from build123d import *

# Parameters (mm, degrees)
SKETCH1_R           = 60
SKETCH1_R_2         = 43.5
EXTRUSION1_DEPTH    = 60
EXTRUSION3_START    = -60
EXTRUSION3_DEPTH    = 60
BOSS_EXTRUDE1_START = -60
BOSS_EXTRUDE1_DEPTH = 60


with BuildPart() as part:
    # Sketch1 → Extrusion1 (new body)
    with BuildSketch(Plane.XY):
        Circle(SKETCH1_R)
        Circle(SKETCH1_R_2, mode=Mode.SUBTRACT)
    extrude(amount=EXTRUSION1_DEPTH)

    # Sketch3 → Extrusion3 (cut)
    with BuildSketch(Plane.XY.offset(60).offset(EXTRUSION3_START)):
        with BuildLine():
            Line((-0.5, 48.5), (-0.5, 43.497126342))
            ThreePointArc((-0.5, 43.497126342), (0, 43.5), (0.5, 43.497126342))
            Line((0.5, 43.497126342), (0.5, 48.5))
            Line((0.5, 48.5), (-0.5, 48.5))
        make_face()
    extrude(amount=EXTRUSION3_DEPTH, mode=Mode.SUBTRACT)

    # Sketch4 → Boss-Extrude1 (add)
    with BuildSketch(Plane.XY.offset(60).offset(BOSS_EXTRUDE1_START)):
        with BuildLine():
            Line((31.28966164, 51.195283713), (31.299038106, 51.211524227))
            Line((31.299038106, 51.211524227), (33.799038106, 55.541651246))
            Line((33.799038106, 55.541651246), (31.200961894, 57.041651246))
            Line((31.200961894, 57.041651246), (28.700961894, 52.711524227))
            Line((28.700961894, 52.711524227), (28.691585429, 52.695283713))
            ThreePointArc((28.691585429, 52.695283713), (30, 51.961524227), (31.28966164, 51.195283713))
        make_face()
        with BuildLine():
            Line((1.5, 59.981247069), (1.5, 60))
            Line((1.5, 60), (1.5, 65))
            Line((1.5, 65), (-1.5, 65))
            Line((-1.5, 65), (-1.5, 60))
            Line((-1.5, 60), (-1.5, 59.981247069))
            ThreePointArc((-1.5, 59.981247069), (0, 60), (1.5, 59.981247069))
        make_face()
        with BuildLine():
            Line((52.695283713, 28.691585429), (52.711524227, 28.700961894))
            Line((52.711524227, 28.700961894), (57.041651246, 31.200961894))
            Line((57.041651246, 31.200961894), (55.541651246, 33.799038106))
            Line((55.541651246, 33.799038106), (51.211524227, 31.299038106))
            Line((51.211524227, 31.299038106), (51.195283713, 31.28966164))
            ThreePointArc((51.195283713, 31.28966164), (51.961524227, 30), (52.695283713, 28.691585429))
        make_face()
        with BuildLine():
            Line((59.981247069, -1.5), (60, -1.5))
            Line((60, -1.5), (65, -1.5))
            Line((65, -1.5), (65, 1.5))
            Line((65, 1.5), (60, 1.5))
            Line((60, 1.5), (59.981247069, 1.5))
            ThreePointArc((59.981247069, 1.5), (60, 0), (59.981247069, -1.5))
        make_face()
        with BuildLine():
            Line((51.195283713, -31.28966164), (51.211524227, -31.299038106))
            Line((51.211524227, -31.299038106), (55.541651246, -33.799038106))
            Line((55.541651246, -33.799038106), (57.041651246, -31.200961894))
            Line((57.041651246, -31.200961894), (52.711524227, -28.700961894))
            Line((52.711524227, -28.700961894), (52.695283713, -28.691585429))
            ThreePointArc((52.695283713, -28.691585429), (51.961524227, -30), (51.195283713, -31.28966164))
        make_face()
        with BuildLine():
            Line((28.691585429, -52.695283713), (28.700961894, -52.711524227))
            Line((28.700961894, -52.711524227), (31.200961894, -57.041651246))
            Line((31.200961894, -57.041651246), (33.799038106, -55.541651246))
            Line((33.799038106, -55.541651246), (31.299038106, -51.211524227))
            Line((31.299038106, -51.211524227), (31.28966164, -51.195283713))
            ThreePointArc((31.28966164, -51.195283713), (30, -51.961524227), (28.691585429, -52.695283713))
        make_face()
        with BuildLine():
            Line((-1.5, -59.981247069), (-1.5, -60))
            Line((-1.5, -60), (-1.5, -65))
            Line((-1.5, -65), (1.5, -65))
            Line((1.5, -65), (1.5, -60))
            Line((1.5, -60), (1.5, -59.981247069))
            ThreePointArc((1.5, -59.981247069), (0, -60), (-1.5, -59.981247069))
        make_face()
        with BuildLine():
            Line((-31.28966164, -51.195283713), (-31.299038106, -51.211524227))
            Line((-31.299038106, -51.211524227), (-33.799038106, -55.541651246))
            Line((-33.799038106, -55.541651246), (-31.200961894, -57.041651246))
            Line((-31.200961894, -57.041651246), (-28.700961894, -52.711524227))
            Line((-28.700961894, -52.711524227), (-28.691585429, -52.695283713))
            ThreePointArc((-28.691585429, -52.695283713), (-30, -51.961524227), (-31.28966164, -51.195283713))
        make_face()
        with BuildLine():
            Line((-52.695283713, -28.691585429), (-52.711524227, -28.700961894))
            Line((-52.711524227, -28.700961894), (-57.041651246, -31.200961894))
            Line((-57.041651246, -31.200961894), (-55.541651246, -33.799038106))
            Line((-55.541651246, -33.799038106), (-51.211524227, -31.299038106))
            Line((-51.211524227, -31.299038106), (-51.195283713, -31.28966164))
            ThreePointArc((-51.195283713, -31.28966164), (-51.961524227, -30), (-52.695283713, -28.691585429))
        make_face()
        with BuildLine():
            Line((-59.981247069, 1.5), (-60, 1.5))
            Line((-60, 1.5), (-65, 1.5))
            Line((-65, 1.5), (-65, -1.5))
            Line((-65, -1.5), (-60, -1.5))
            Line((-60, -1.5), (-59.981247069, -1.5))
            ThreePointArc((-59.981247069, -1.5), (-60, 0), (-59.981247069, 1.5))
        make_face()
        with BuildLine():
            Line((-51.195283713, 31.28966164), (-51.211524227, 31.299038106))
            Line((-51.211524227, 31.299038106), (-55.541651246, 33.799038106))
            Line((-55.541651246, 33.799038106), (-57.041651246, 31.200961894))
            Line((-57.041651246, 31.200961894), (-52.711524227, 28.700961894))
            Line((-52.711524227, 28.700961894), (-52.695283713, 28.691585429))
            ThreePointArc((-52.695283713, 28.691585429), (-51.961524227, 30), (-51.195283713, 31.28966164))
        make_face()
        with BuildLine():
            Line((-28.691585429, 52.695283713), (-28.700961894, 52.711524227))
            Line((-28.700961894, 52.711524227), (-31.200961894, 57.041651246))
            Line((-31.200961894, 57.041651246), (-33.799038106, 55.541651246))
            Line((-33.799038106, 55.541651246), (-31.299038106, 51.211524227))
            Line((-31.299038106, 51.211524227), (-31.28966164, 51.195283713))
            ThreePointArc((-31.28966164, 51.195283713), (-30, 51.961524227), (-28.691585429, 52.695283713))
        make_face()
    extrude(amount=BOSS_EXTRUDE1_DEPTH)


solid = part.part
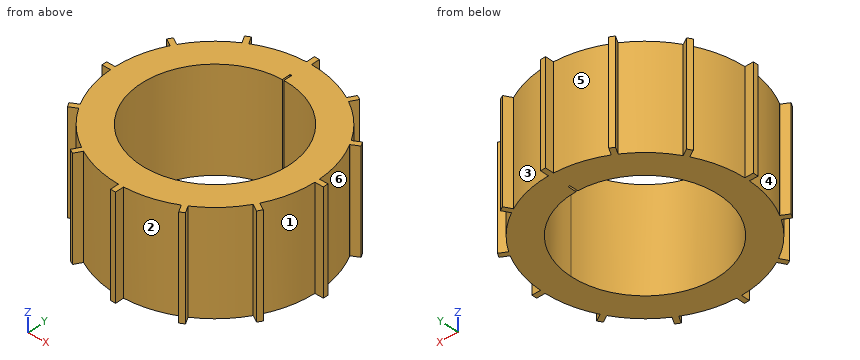
Source: CAD feature listing. Evaluate the final solid. Frame: model axes, mm. Face numbers are marked on the shaded views. A direction names the side the tool comes from. Round coordinates to 2 decimals unless told otherwise and drop trailing zeros. Write each loop counter-clockwise with the first axis right and the second up, starting at its lowest first coordinate (ties: lowest second). Pieces come first, ordered by that corner, then holes. Notation, with made-up numbers: (52.5, -2) - (61.5, -2) arc R19 ccw to (61.5, 25) - close; hole circle Ø5 at (53.25, -27.5). An arc over 180 degrees is marked (long way). Use CSV: the item, a comma, the result in double quotes. Start each with the question number.
(1) Cut plane B-B, the plane y = 10. Return loops of the section in (x, z).
(2) Cut plane A-A, the plane x = 23. Return loops of the section in (y, z).
(3) Mould query, pull axis X, two halves, no side actions, for the marked faces 4, 5 and 6. Classes: pulls with the +X half, pulls with the -X half, needs draft (parallel to the pull), parting line crosses it, or undercut.
(4) First-contact query: pin 1 Ø1 at (x, z) = (42.5, 26) entering from -Y; pin 2 Ø5.5 at (y, z) = (45.5, 42) entering from -X; pin 3 Ø5.5 at (x, z) = (63.5, 38) entering from -Y. Flat tips, straight axial feed; report the tip coordinate or a pass-through.
(5) Set-up query: the marked faces 1, 2 and 3. Return all of +Z, -Z, +X, -X, +Y, -Y with unobstructed straight access to the full face (end or side cutting, diameter ignored); none if empty.
(6) Material intervals for probe 1 along X at (y, z) = (0, 20.5); probe 2 along Y at (x, z) = (0, 39); probe 3 along X at (y, z) = (-36.5, 37), sorted ascending. Write a range as [from, to].
Geometry says:
1,outline,"(-59.16, 0) - (-42.33, 0) - (-42.33, 60) - (-59.16, 60) - close; (42.33, 0) - (59.16, 0) - (59.16, 60) - (42.33, 60) - close"
2,outline,"(-55.42, 0) - (-36.92, 0) - (-36.92, 60) - (-55.42, 60) - close; (36.92, 0) - (55.42, 0) - (55.42, 60) - (36.92, 60) - close"
3,face 4,"pulls with the -X half"
3,face 5,"undercut"
3,face 6,"pulls with the +X half"
4,pin 1,"y = -42.85"
4,pin 2,"x = -42.1"
4,pin 3,"y = -1.5"
5,face 1,"+Z, -Z, +X"
5,face 2,"+Z, -Z, -Y"
5,face 3,"+Z, -Z, +Y"
6,probe 1,"[-65, -43.5], [43.5, 65]"
6,probe 2,"[-65, -43.5], [48.5, 65]"
6,probe 3,"[-47.62, -23.66], [23.66, 47.62]"
